Work out the finished part from the listing and answer in its coordinate system (mm). Face numbers are marked on the shaded views. A direction names the side the tool comes from. Round coordinates to 2 decimals unless told otherwise and drop trailing zeros. Write each loop counter-clockwise with the first axis right and the second up, starting at its lowest first coordinate (ties: lowest second). Pieces come first, ordered by that corner, then holes. Notation, with made-up numbers: M 58.5,49 L 72.5,49 A19 ccw 72.5,78 Z; hole C 46,19.25 d2. An arc over 180 degrees is marked long. One line per item, written item: value. Start each with the question number.
Q1. Find section A-A (z = -5.25). Write down the section's boundary in (x, y).
Q2. A tool of negligible diameter and unlimited length cuts with its end or side. For the marked faces 4 and 5, from which of +Z, -Z, +X, -X, +Y, -Y can it reach the whole face along a straight path? Write none if from no direction.
Q3. The mould has two halves that part along Y. Classify the marked faces 1, 2 and 3: released by +Y, released by -Y, zero draft, split by the parting line, or undercut.
Q4. Given pin 1 Ø3 at (y, z) = (-1, -5) entering from +X; pin 2 Ø5 at (x, z) = (-2, -7) entering from -Y; pin 3 Ø8 at (y, z) = (1, -14.5) entering from -X, each flat-ended and moving along its own axis, determine where each tip first touches the part or whether it passes through.
Q5. Consider probe 1 along Z at (x, y) = (2.25, -1.25); probe 2 along Y at (x, z) = (0.25, -2.5); probe 3 along Y at (x, z) = (0.75, -17). Determine where each line is inside the solid, lowest interval first.
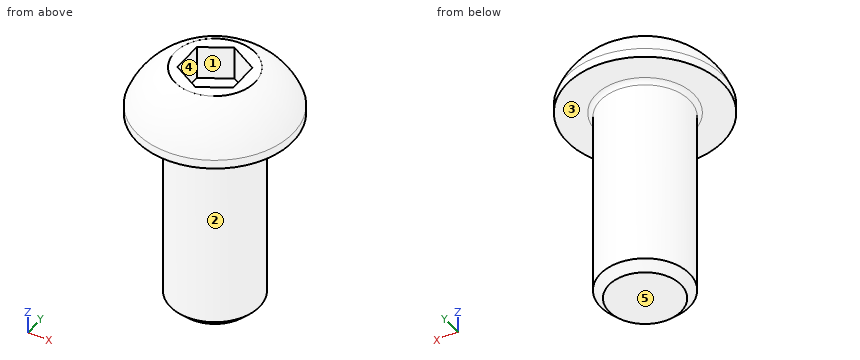
from build123d import *

# Parameters (mm, degrees)
SKETCH2_R           = 4
BOSS_EXTRUDE1_DEPTH = 18
CUT_EXTRUDE1_DEPTH  = 3
CHAMFER1_SIZE       = 0.7668
FILLET1_R           = 0.4


with BuildPart() as part:
    # Sketch1 → Revolve1 (revolve)
    with BuildSketch(Plane.XZ, mode=Mode.PRIVATE) as revolve1_sk:
        with BuildLine():
            Line((3.603028, 4.4), (0, 4.4))
            Line((0, 4.4), (0, 0))
            Line((0, 0), (7, 0))
            Line((7, 0), (7, 0.8))
            ThreePointArc((7, 0.8), (5.673259557, 2.950780347), (3.603028, 4.4))
        make_face()
    revolve(revolve1_sk.sketch.rotate(Axis((0, 0, 4.4), (0, 0, -1)), 180), axis=Axis((0, 0, 4.4), (0, 0, -1)))

    # Sketch2 → Boss-Extrude1 (add)
    with BuildSketch(Plane(origin=(0, 0, 0), x_dir=(-1, 0, 0), z_dir=(0, 0, -1))):
        Circle(SKETCH2_R)
    extrude(amount=BOSS_EXTRUDE1_DEPTH)

    # Sketch3 → Cut-Extrude1 (cut)
    with BuildSketch(Plane.XY.offset(4.4)):
        Polygon((2.5, -1.443375673), (2.5, 1.443375673), (0, 2.886751346), (-2.5, 1.443375673), (-2.5, -1.443375673), (0, -2.886751346), align=None)
    extrude(amount=-CUT_EXTRUDE1_DEPTH, mode=Mode.SUBTRACT)

    # Chamfer1
    chamfer1_edges = [part.edges().sort_by_distance(p)[0] for p in [
        (4, 0, -18),
    ]]
    chamfer(chamfer1_edges, length=CHAMFER1_SIZE)

    # Fillet1
    fillet1_edges = [part.edges().sort_by_distance(p)[0] for p in [
        (4, 0, 0),
    ]]
    fillet(fillet1_edges, radius=FILLET1_R)


solid = part.part
The answers:
1. outline: C 0,0 d8
2. face 4: +Z
2. face 5: -Z, +X, -X, +Y, -Y
3. face 1: undercut
3. face 2: split by the parting line
3. face 3: zero draft
4. pin 1: x = 4
4. pin 2: y = -4
4. pin 3: x = -4
5. probe 1: -18 to 1.4
5. probe 2: -3.99 to 3.99
5. probe 3: -3.93 to 3.93
